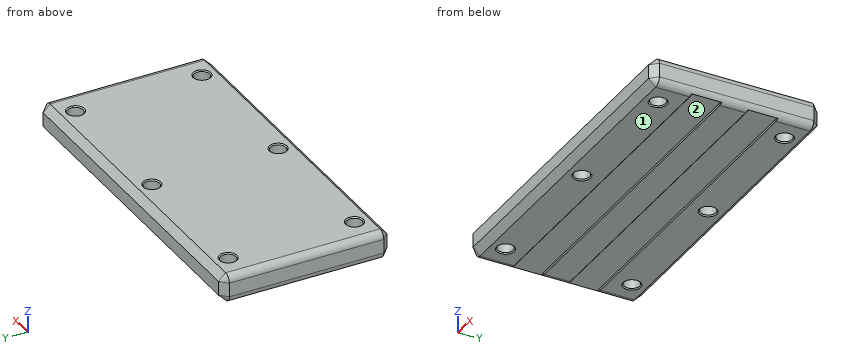
from build123d import *

# Parameters (mm, degrees)
SKETCH1_W                     = 76.2
SKETCH1_H                     = 38.1
BOSS_EXTRUDE1_DEPTH           = 3.175
SKETCH1_2_W                   = 76.2
SKETCH1_2_H                   = 38.1
BOSS_EXTRUDE2_DEPTH           = 3.175
SKETCH10_W                    = 76.2
SKETCH10_H                    = 6.35
CUT_EXTRUDE2_DEPTH            = 0.254
M3_CLEARANCE_HOLE1_AT_2_COUNT = 2
M3_CLEARANCE_HOLE1_AT_2_PITCH = 28.575
M3_CLEARANCE_HOLE1_AT_3_COUNT = 2
M3_CLEARANCE_HOLE1_AT_3_PITCH = 31.75
M3_CLEARANCE_HOLE1_AT_4_COUNT = 2
M3_CLEARANCE_HOLE1_AT_4_PITCH = 42.715256349
M3_CLEARANCE_HOLE1_AT_5_COUNT = 2
M3_CLEARANCE_HOLE1_AT_5_PITCH = 63.5
M3_CLEARANCE_HOLE1_AT_6_COUNT = 2
M3_CLEARANCE_HOLE1_AT_6_PITCH = 69.633186233
FILLET1_R                     = 1.5875
CHAMFER1_SIZE                 = 1.5875
CHAMFER3_SIZE                 = 0.254


with BuildPart() as part:
    # Sketch1 → Boss-Extrude1 (new, symmetric)
    with BuildSketch(Plane.XY):
        Rectangle(SKETCH1_W, SKETCH1_H)
    extrude(amount=BOSS_EXTRUDE1_DEPTH, both=True)

    # Sketch1<2> → Boss-Extrude2 (add, symmetric)
    with BuildSketch(Plane.XY):
        Rectangle(SKETCH1_2_W, SKETCH1_2_H)
    extrude(amount=BOSS_EXTRUDE2_DEPTH, both=True)

    # Sketch10 → Cut-Extrude2 (cut)
    with BuildSketch(Plane(origin=(0, 0, -3.175), x_dir=(-1, 0, 0), z_dir=(0, 0, -1))):
        with Locations((0, 6.35)):
            Rectangle(SKETCH10_W, SKETCH10_H)
        with Locations((0, -6.35)):
            Rectangle(SKETCH10_W, SKETCH10_H)
    extrude(amount=-CUT_EXTRUDE2_DEPTH, mode=Mode.SUBTRACT)

    # Sketch4 → M3 Clearance Hole1 (revolve, cut)
    with BuildSketch(Plane(origin=(-31.75, 14.2875, 3.175), x_dir=(0, -1, 0), z_dir=(1, 0, 0))):
        Polygon((0, 0), (0, 6.35), (2, 6.35), (1.75, 6.1), (1.75, 0.25), (2, 0), align=None)
    m3_clearance_hole1 = revolve(axis=Axis((-31.75, 14.2875, 9.525), (0, 0, -1)), mode=Mode.SUBTRACT)

    # M3 Clearance Hole1 at 2: M3 Clearance Hole1 ×2
    with Locations(*[(0, -i * M3_CLEARANCE_HOLE1_AT_2_PITCH, 0) for i in range(1, M3_CLEARANCE_HOLE1_AT_2_COUNT)]):
        add(m3_clearance_hole1, mode=Mode.SUBTRACT)

    # M3 Clearance Hole1 at 3: M3 Clearance Hole1 ×2
    with Locations(*[(i * M3_CLEARANCE_HOLE1_AT_3_PITCH, 0, 0) for i in range(1, M3_CLEARANCE_HOLE1_AT_3_COUNT)]):
        add(m3_clearance_hole1, mode=Mode.SUBTRACT)

    # M3 Clearance Hole1 at 4: M3 Clearance Hole1 ×2
    with Locations(*[Vector(0.7432941462471665, -0.6689647316224495, 0) * (i * M3_CLEARANCE_HOLE1_AT_4_PITCH) for i in range(1, M3_CLEARANCE_HOLE1_AT_4_COUNT)]):
        add(m3_clearance_hole1, mode=Mode.SUBTRACT)

    # M3 Clearance Hole1 at 5: M3 Clearance Hole1 ×2
    with Locations(*[(i * M3_CLEARANCE_HOLE1_AT_5_PITCH, 0, 0) for i in range(1, M3_CLEARANCE_HOLE1_AT_5_COUNT)]):
        add(m3_clearance_hole1, mode=Mode.SUBTRACT)

    # M3 Clearance Hole1 at 6: M3 Clearance Hole1 ×2
    with Locations(*[Vector(0.9119215051751064, -0.4103646773287979, 0) * (i * M3_CLEARANCE_HOLE1_AT_6_PITCH) for i in range(1, M3_CLEARANCE_HOLE1_AT_6_COUNT)]):
        add(m3_clearance_hole1, mode=Mode.SUBTRACT)

    # Fillet1
    fillet1_edges = [part.edges().sort_by_distance(p)[0] for p in [
        (-38.1, -14.2875, -3.175),
        (-38.1, 0, 3.175),
        (38.1, 0, 3.175),
        (38.1, -14.2875, -3.175),
    ]]
    fillet(fillet1_edges, radius=FILLET1_R)

    # Chamfer1
    chamfer1_edges = [part.edges().sort_by_distance(p)[0] for p in [
        (-38.1, -19.05, 0),
        (-38.1, 19.05, 0),
        (0, -19.05, -3.175),
        (38.1, -19.05, 0),
        (0, -19.05, 3.175),
        (37.635032015, -19.05, -2.710032015),
        (37.635032015, -19.05, 2.710032015),
        (-37.635032015, -19.05, 2.710032015),
        (-37.635032015, -19.05, -2.710032015),
        (-2.84e-07, 19.05, -3.175),
        (0, 19.05, 3.175),
        (38.1, 19.05, 0),
        (37.635032015, 19.05, -2.710032015),
        (37.635032015, 19.05, 2.710032015),
        (-37.635032015, 19.05, 2.710032015),
        (-37.635032216, 19.05, -2.710031814),
    ]]
    chamfer(chamfer1_edges, length=CHAMFER1_SIZE)

    # Chamfer3
    chamfer3_edges = [part.edges().sort_by_distance(p)[0] for p in [
        (0, -9.525, -3.175),
        (36.961512806, -9.525, -3.110176509),
        (-36.961512806, -9.525, -3.110176509),
        (2.84e-07, -3.175, -3.175),
        (36.961513079, -3.175, -3.110176428),
        (-36.961512806, -3.175, -3.110176509),
        (-2.84e-07, 3.175, -3.175),
        (36.961512806, 3.175, -3.110176509),
        (-36.961513079, 3.175, -3.110176428),
        (2.84e-07, 9.525, -3.175),
        (36.961513079, 9.525, -3.110176428),
        (-36.961512806, 9.525, -3.110176509),
    ]]
    chamfer(chamfer3_edges, length=CHAMFER3_SIZE - 0.0001)  # a hair under: the kernel refuses the full size


solid = part.part
Can you work these out from the model? Positions are in its coordinate system, mm. Face numbers are marked on the shaded views. A direction names the side the tool comes from. Give positions to 0.01 mm unless a question says otherwise; leave off trailing zeros. Loops run counter-clockwise (first coordinate to the right, second up) from the corner with the lowest first, then second, coordinate; pieces in that order, holes last. Notation, with made-up numbers: M 60.5,-32 L 70.5,-32 A14 ccw 70.5,-19 Z; hole C 74.25,76.5 d7. An arc over 180 degrees is marked long. One line per item, written item: value. Start each with the question number.
1) I'm going to push flat-ended pins straight in: pin 1 (5.5 mm diameter, centred on x = -31.75, y = 14.29, fed in from +Z) (3 decimals); pin 2 (3 mm diameter, centred on x = 0, y = 14.29, fed in from +Z); pin 3 (1.5 mm diameter, centred on x = -7, z = -2.5, fed in from +Y). Where does each tip first touch, or does it pass through?
2) If we section it at D-D, the plane x = 0: Give the number of separate pieces and of enclosed holes in the cut face, and give its area (3 significant figures).
3) If we section it at B-B, the plane z = 0.5: Write out the boundary of the cut face in (x, y).
4) On a 3-axis mill with a long thin cutter (end or side, diameter ignored), from which of +Z, -Z, +X, -X, +Y, -Y can I reach the whole of each face in a straight line? I mean the marked faces 1 and 2. Say none if no direction works.
5) If we section it at C-C, the plane y = -6.5: Write out the boundary of the cut face in (x, z) (1 decimal), and give its area (3 significant figures).
6) If I drill on line 1 (Y direction, x = -31.75, z = -1.1); line 2 (X direction, y = -15.5, z = 2.75); line 3 (X direction, y = -13, z = -1.5), over which ranges is the centre line in solid material (lowest first)? Write a range as [from, to].
Completed:
1. pin 1: stops at z = 3.175
1. pin 2: passes through
1. pin 3: stops at y = 18.89
2. separate pieces: 3
2. enclosed holes: 0
2. area: 189 mm^2
3. outline: M -38.1,-17.46 L -36.51,-19.05 L 36.51,-19.05 L 38.1,-17.46 L 38.1,17.46 L 36.51,19.05 L -36.51,19.05 L -38.1,17.46 Z; hole C -31.75,-14.29 d3.5; hole C -31.75,14.29 d3.5; hole C 0,-14.29 d3.5; hole C 0,14.29 d3.5; hole C 31.75,-14.29 d3.5; hole C 31.75,14.29 d3.5
4. face 1: -Z, +X, -X, +Y, -Y
4. face 2: -Z, +X, -X
5. outline: M -38.1,-1.6 A1.6 ccw -37.4,-2.9 L 37.4,-2.9 A1.6 ccw 38.1,-1.6 L 38.1,1.6 A1.6 ccw 36.5,3.2 L -36.5,3.2 A1.6 ccw -38.1,1.6 Z
5. area: 463 mm^2
6. line 1: y = [-19.05, -16.04], [-12.54, 12.54], [16.04, 19.05]
6. line 2: x = [-37.59, -33.01], [-30.49, -1.26], [1.26, 30.49], [33.01, 37.59]
6. line 3: x = [-38.1, -32.94], [-30.56, -1.19], [1.19, 30.56], [32.94, 38.1]
